Input: part model. Units: mm. Frame: model coordinates. Face numbers are marked on the shaded views. A direction names the side the tool comes from. Coordinates: 2 decimals unless noted, no trailing zeros. Write each loop counter-clockwise with the first axis right and the second up, starting at its lowest first coordinate (ties: lowest second). Pieces come first, ordered by that corner, then holes. Notation, with made-up numbers: M 30,76.25 L 43,76.25 A10 ccw 43,91.25 Z; hole C -7,52 d9. An arc over 180 degrees is marked long. Answer as a JSON object with one key per item and string values. Group by question number.
from build123d import *

# Parameters (mm, degrees)
SKETCH_1_W          = 20
SKETCH_1_H          = 20
EXTRUDE_1_DEPTH     = 5
SKETCH_3_W          = 20
SKETCH_3_H          = 80
SKETCH_3_W_2        = 15
SKETCH_3_H_2        = 45
EXTRUDE_2_DEPTH     = 2.5
FILLET_1_R          = 10
SKETCH_5_R          = 4
CUT_EXTRUDE_1_DEPTH = 82.58584436
SKETCH_6_R          = 6
EXTRUDE_3_DEPTH     = 6


with BuildPart() as part:
    # 草图1 → 凸台-拉伸1 (new body)
    with BuildSketch(Plane.XY):
        Rectangle(SKETCH_1_W, SKETCH_1_H)
    extrude(amount=EXTRUDE_1_DEPTH)

    # 草图3 → 凸台-拉伸2 (add, symmetric)
    with BuildSketch(Plane(origin=(0, 0, 0), x_dir=(1, 0, 0), z_dir=(0, 1, 0))):
        with Locations((0, 40)):
            Rectangle(SKETCH_3_W, SKETCH_3_H)
        with Locations((0, 27.5)):
            Rectangle(SKETCH_3_W_2, SKETCH_3_H_2, mode=Mode.SUBTRACT)
    extrude(amount=EXTRUDE_2_DEPTH, both=True)

    # 圆角1
    fillet_1_edges = [part.edges().sort_by_distance(p)[0] for p in [
        (10, 0, -80),
        (-10, 0, -80),
    ]]
    fillet(fillet_1_edges, radius=FILLET_1_R - 0.0001)  # a hair under: the kernel refuses the full size

    # 草图5 → 切除-拉伸1 (cut, through all)
    with BuildSketch(Plane(origin=(0, 2.5, 0), x_dir=(1, 0, 0), z_dir=(0, 1, 0))):
        with Locations(Location((0, 70, 0), (0, 0, 270))):
            Circle(SKETCH_5_R)
    extrude(amount=-CUT_EXTRUDE_1_DEPTH, mode=Mode.SUBTRACT)

    # 草图6 → 凸台-拉伸3 (add, symmetric)
    with BuildSketch(Plane(origin=(0, 0, 0), x_dir=(1, 0, 0), z_dir=(0, 1, 0))):
        with BuildLine():
            Line((-10, -5), (-10, -15))
            ThreePointArc((-10, -15), (0, -25), (10, -15))
            Line((10, -15), (10, -5))
            Line((10, -5), (-10, -5))
        make_face()
        with Locations(Location((0, -15, 0), (0, 0, 270))):
            Circle(SKETCH_6_R, mode=Mode.SUBTRACT)
    extrude(amount=EXTRUDE_3_DEPTH, both=True)


solid = part.part
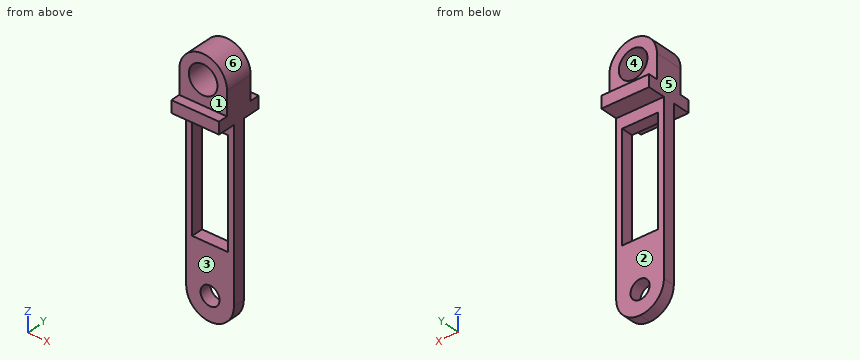
Q1. Access query for the marked faces 1, 2 and 3. Directions: +Z, -Z, +X, -X, +Y, -Y. A direction counts if a zero-diameter tool reaches every point of the face in a straight line with its end or side. Return the directions, or none.
Q2. Section B-B, the plane y = 4.5. Return the cut outline in (x, z), and give its area (3 significant figures).
Q3. Draft query along Z for the marked faces 4, 5 and 6. Return one class per face: released by +Z, released by -Z, zero draft, split by the parting line, or undercut.
Q4. Section A-A, the plane z = -35.5. Return the cut outline in (x, y).
Q5. Pin query (flat end, axial travel): pin 1 Ø9 at (x, z) = (0, -70) entering from +Y; pin 2 Ø3 at (x, y) = (-1.5, 9) entering from +Z; pin 3 Ø2 at (x, y) = (-3.5, 6.5) entering from -Z. Return the tip coordinate at first contact, or that it passes through.
Q6. Line query: line 1 (X direction, y = 0.15, z = -70); line 2 (X direction, y = -1, z = 15); line 3 (Y direction, x = 9.25, z = -62.5). Output: solid intervals per line, ascending. Write a range as from..to.
Q7. Section C-C, the plane y = -8.5. Return the cut outline in (x, z).
Filled in:
{
 "1": {"face 1": "+Z, +X, -X, -Y", "face 2": "-Z, +X, -X, +Y", "face 3": "-Z, +X, -X, -Y"},
 "2": {"outline": "M -10,0 L 10,0 L 10,15 A10 ccw -10,15 Z; hole C 0,15 d12", "area": "344 mm^2"},
 "3": {"face 4": "undercut", "face 5": "zero draft", "face 6": "released by +Z"},
 "4": {"outline": "M -10,-2.5 L -7.5,-2.5 L -7.5,2.5 L -10,2.5 Z; M 7.5,-2.5 L 10,-2.5 L 10,2.5 L 7.5,2.5 Z"},
 "5": {"pin 1": "y = 2.5", "pin 2": "z = 5", "pin 3": "z = 0"},
 "6": {"line 1": "-10..-4, 4..10", "line 2": "-10..-6, 6..10", "line 3": "-2.5..2.5"},
 "7": {"outline": "M -10,0 L 10,0 L 10,5 L -10,5 Z"}
}
